Build history of the part. All positions in model axes, mm. Round coordinates to 2 decimals unless told otherwise and drop trailing zeros. Loops run counter-clockwise (first coordinate to the right, second up) from the corner with the lowest first, then second, coordinate; pieces in that order, holes last. Notation, with made-up numbers: M 80,2 L 136,2 A20 cw 136,38 Z; hole C -3.5,37 d6. An arc over 180 degrees is marked long. One line per item, written item: value.
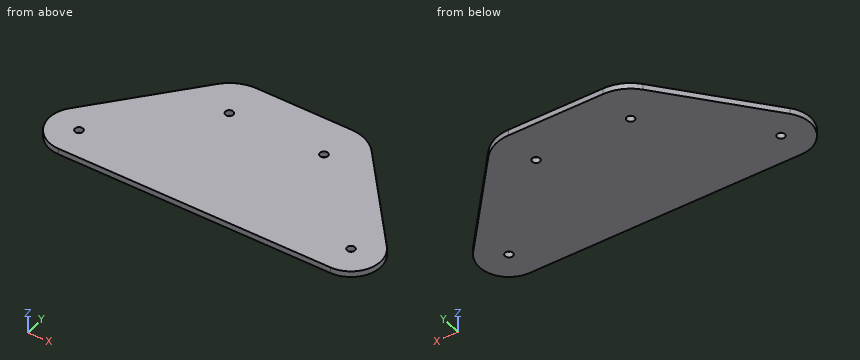
Autodesk Inventor part; units mm, degrees
ref_plane "YZ Plane" through (0, 0, 0) normal (1, 0, 0) x (0, 1, 0)
ref_plane "XZ Plane" through (0, 0, 0) normal (0, 1, 0) x (-1, 0, 0)
ref_plane "XY Plane" through (0, 0, 0) normal (0, 0, 1) x (1, 0, 0)
sketch "Sketch1" plane through (0, 0, 0) normal (0, 0, 1) x (1, 0, 0)
  line L0 (0, 80) -> (0, 0)
  line L1 (0, 80) -> (24, 80)
  arc A0 (39.2095, 72.9873) -> (24, 80) centre (24, 60) ccw
  line L2 (39.2095, 72.9873) -> (80.4071, 24.7405)
  arc A1 (69, 0) -> (80.4071, 24.7405) centre (69, 15) ccw
  line L3 (69, 0) -> (0, 0)
  circle A2 centre (24, 60) radius 2
  circle A3 centre (69, 15) radius 2
  dimension "d0" = 24
  dimension "d1" = 20
  dimension "d2" = 45
  dimension "d3" = 45
  dimension "d4" = 15
  dimension "d5" = 4
  dimension "d6" = 4
extrude "Extrusion1" add sketch "Sketch1" along normal blind 3
mirror "Mirror1" about plane through (0, 0, 0) normal (1, 0, 0) of "Extrusion1"
equation "\"d3\" = d2"
properties part number "clawBase"
Item 1: Slice it at C-C, the plane y = 60. Give the cut face in (x, z), and give its area (3 significant figures).
Check values:
outline: M -50.3,0 L -26,0 L -26,3 L -50.3,3 Z; M -22,0 L 22,0 L 22,3 L -22,3 Z; M 26,0 L 50.3,0 L 50.3,3 L 26,3 Z
area: 278 mm2
Item 2: Slice it at A-A, the plane y = 15. Give the cut face in (x, z), and give its area (3 significant figures).
Check values:
outline: M -84,0 L -71,0 L -71,3 L -84,3 Z; M -67,0 L 67,0 L 67,3 L -67,3 Z; M 71,0 L 84,0 L 84,3 L 71,3 Z
area: 480 mm2
Item 3: Slice it at D-D, the plane y = 6. Give the cut face in (x, z), and give its area (3 significant figures).
Check values:
outline: M -81,0 L 81,0 L 81,3 L -81,3 Z
area: 486 mm2
Item 4: Wall check: line 1 along X through (y, z) = (61.5, 0.8); line 2 along Y through (x, z) = (-24, 0.95); line 3 along Y through (x, z) = (69, 2.15). Give the ranges that are in metal, low to high.
Check values:
line 1: x = -49.02 to -25.32, -22.68 to 22.68, 25.32 to 49.02
line 2: y = 0 to 58, 62 to 80
line 3: y = 0 to 13, 17 to 38.1
Item 5: Slice it at B-B, the plane z = 0.9. Give the cut face in (x, y).
Check values:
outline: M -80.41,24.74 A15 ccw -69,0 L 69,0 A15 ccw 80.41,24.74 L 39.21,72.99 A20 ccw 24,80 L -24,80 A20 ccw -39.21,72.99 Z; hole C -69,15 d4; hole C -24,60 d4; hole C 24,60 d4; hole C 69,15 d4
Item 6: Drop a flat-ended pin along its axis: P1, Ø1.5, axis at y = 10, z = 2.5, coming from the -X side. Give the stop position or say it passes through.
Check values:
P1: stops at x = -83.39
